The model under review builds one solid part; all positions refer to its coordinate system, in mm. A direction names the side the tool comes from. Coordinates: 2 decimals unless noted, no trailing zeros. Order: outer loops, then holes, each group sorted by start corner. A loop starts at its lowest first (then second) coordinate and runs counter-clockwise, first axis right, second up. Notation, with made-up numbers: M -13,3 L -6,3 A24 cw -6,24 Z; hole C 63.5,82 d3. An arc over 180 degrees is marked long. One line per item, written item: value.
```python
from build123d import *

# Parameters (mm, degrees)
SKETCH1_W           = 30
SKETCH1_H           = 20
BOSS_EXTRUDE1_DEPTH = 5
SKETCH2_R           = 3
CUT_EXTRUDE1_DEPTH  = 10
SKETCH3_OUTSIDE_W   = 39.28
SKETCH3_OUTSIDE_H   = 29.28
SKETCH3_OUTSIDE_W_2 = 24.327904035
SKETCH3_OUTSIDE_H_2 = 11.132815548
CUT_EXTRUDE2_DEPTH  = 10
SKETCH4_W           = 11.132815548
SKETCH4_H           = 20
BOSS_EXTRUDE2_DEPTH = 5
SKETCH5_R           = 1.6
CUT_EXTRUDE3_DEPTH  = 5
FILLET2_R           = 5


with BuildPart() as part:
    # Sketch1 → Boss-Extrude1 (new body)
    with BuildSketch(Plane(origin=(0, 0, 0), x_dir=(1, 0, 0), z_dir=(0, 1, 0))):
        Rectangle(SKETCH1_W, SKETCH1_H)
    extrude(amount=BOSS_EXTRUDE1_DEPTH)

    # Sketch2 → Cut-Extrude1 (cut)
    with BuildSketch(Plane(origin=(0, 5, 0), x_dir=(1, 0, 0), z_dir=(0, 1, 0))):
        with Locations(Location((0, 0, 0), (0, 0, 270))):
            Circle(SKETCH2_R)
    extrude(amount=-CUT_EXTRUDE1_DEPTH, mode=Mode.SUBTRACT)

    # Sketch3 outside → Cut-Extrude2 (cut)
    with BuildSketch(Plane(origin=(0, 5, 0), x_dir=(1, 0, 0), z_dir=(0, 1, 0))):
        Rectangle(SKETCH3_OUTSIDE_W, SKETCH3_OUTSIDE_H)
        with Locations((-2.836047983, 0)):
            Rectangle(SKETCH3_OUTSIDE_W_2, SKETCH3_OUTSIDE_H_2, mode=Mode.SUBTRACT)
    extrude(amount=-CUT_EXTRUDE2_DEPTH, mode=Mode.SUBTRACT)

    # Sketch4 → Boss-Extrude2 (add)
    with BuildSketch(Plane.ZY.offset(15)):
        with Locations((0, 2.5)):
            Rectangle(SKETCH4_W, SKETCH4_H)
    extrude(amount=BOSS_EXTRUDE2_DEPTH)

    # Sketch5 → Cut-Extrude3 (cut)
    with BuildSketch(Plane.ZY.offset(20)):
        with Locations((0, 9)):
            Circle(SKETCH5_R)
        with Locations(Location((0, -4, 0), (0, 0, 180))):
            Circle(SKETCH5_R)
    extrude(amount=-CUT_EXTRUDE3_DEPTH, mode=Mode.SUBTRACT)

    # Fillet2
    fillet2_edges = [part.edges().sort_by_distance(p)[0] for p in [
        (9.327904035, 2.5, -5.566407774),
        (9.327904035, 2.5, 5.566407774),
    ]]
    fillet(fillet2_edges, radius=FILLET2_R)


solid = part.part
```
(1) We need section A-A, the plane y = 9. State the section outline as (x, z) points, plus the area to 3 significant figures.
Geometry results:
outline: M -20,-5.57 L -15,-5.57 L -15,-1.6 L -20,-1.6 Z; M -20,1.6 L -15,1.6 L -15,5.57 L -20,5.57 Z
area: 39.7 mm2
(2) Tool access review of faces 4 (the flat face through (-3, 0, -1)), 5 (the flat face through (-20, 3, 0)), 6 (the flat face through (-15, 7, 0)): name each direction out of +Z, -Z, +X, -X, +Y, -Y from which nothing blocks a thin tool from reaching the whole face with its end or side.
Geometry results:
face 4: +Z, -Z, +X, -Y
face 5: +Z, -Z, -X, +Y, -Y
face 6: +Z, -Z, +X, +Y
(3) We need section B-B, the plane x = 0. State the section outline as (y, z) points.
Geometry results:
outline: M 0,-5.57 L 5,-5.57 L 5,-3 L 0,-3 Z; M 0,3 L 5,3 L 5,5.57 L 0,5.57 Z
(4) Mouldability with a two-part tool opening along Z and no side actions: class faces 1 (the cylindrical face through (0.9, 2.54, 2.86)), 2 (the flat face through (-15, -2, 0)), 3 (the cylindrical face through (7.824, 2.465, -4.141)) as +Z half, -Z half, draft (parallel to the pull), parting line (faces both ways), or undercut.
Geometry results:
face 1: undercut
face 2: draft
face 3: -Z half
(5) Insertion check: pin 1 Ø2 at (y, z) = (2, -3.5) entering from +X; pin 2 Ø4 at (y, z) = (7.5, -2) entering from +X; pin 3 Ø1 at (x, z) = (2, 4) entering from -Y. Each pin has a flat end and moves straight along its axis. Give the tip position at first contact, or say it passes through.
Geometry results:
pin 1: stops at x = 8.94
pin 2: stops at x = -15
pin 3: stops at y = 0
(6) For L1, parallel to Y at x = -17.15, z = 0; L2, parallel to X at y = 2.35, z = 0; L3, parallel to Z at x = -17.15, y = -4, list the stretches that pass through material, from the lowest coordinate up.
Geometry results:
L1: y = -7.5 to -5.6, -2.4 to 7.4, 10.6 to 12.5
L2: x = -20 to -3, 3 to 9.33
L3: z = -5.57 to -1.6, 1.6 to 5.57
(7) We need section D-D, the plane y = 1.75. State the section outline as (x, z) points.
Geometry results:
outline: M -20,-5.57 L 4.33,-5.57 A5 ccw 9.33,-0.57 L 9.33,0.57 A5 ccw 4.33,5.57 L -20,5.57 Z; hole C 0,0 d6
(8) We need section C-C, the plane z = 0. State the section outline as (x, y) points.
Geometry results:
outline: M -20,-7.5 L -15,-7.5 L -15,-5.6 L -20,-5.6 Z; M -20,-2.4 L -15,-2.4 L -15,0 L -3,0 L -3,5 L -15,5 L -15,7.4 L -20,7.4 Z; M -20,10.6 L -15,10.6 L -15,12.5 L -20,12.5 Z; M 3,0 L 9.33,0 L 9.33,5 L 3,5 Z
